Geometry: final body of the model. Coordinates: model frame, mm. A direction names the side the tool comes from. Give positions to 0.01 mm unless a question says otherwise; leave off trailing zeros. Loops run counter-clockwise (first coordinate to the right, second up) from the corner with the lowest first, then second, coordinate; pieces in that order, holes last. Notation, with made-up numbers: (35.25, 23) - (88.25, 23) arc R16 cw to (88.25, 31) - close; hole circle Ø2 at (73.5, 86.25). An arc over 180 degrees is marked (long way). Answer in a Markdown table with one row per item.
from build123d import *

# Parameters (mm, degrees)
F1_DEPTH = 5
F3_DEPTH = 22
F5_D     = 12
F5_DEPTH = 24
F5_TIP   = 3.6051637142
F7_D     = 6
F7_DEPTH = 16
F7_TIP   = 1.8025818571


with BuildPart() as f1:
    # F0 (on Front) → F1 (new body, symmetric)
    with BuildSketch(Plane.XZ):
        Polygon((32, -18), (32, 18), (-32, 18), (-32, -18), (-8, -18), (-8, -27), (8, -27), (8, -18), align=None)
    extrude(amount=F1_DEPTH, both=True)

    # F2 (on face) → F3 (join)
    with BuildSketch(Plane.XZ.offset(5)):
        with BuildLine():
            Line((-27.5, -8), (-32, -8))
            Line((-32, -8), (-32, -18))
            Line((-32, -18), (-8, -18))
            Line((-8, -18), (-8, -27))
            Line((-8, -27), (8, -27))
            Line((8, -27), (8, -18))
            Line((8, -18), (32, -18))
            Line((32, -18), (32, -8))
            Line((32, -8), (27.5, -8))
            ThreePointArc((27.5, -8), (26.0843309615, -7.6449728115), (25.0037292554, -6.6639207823))
            Line((25.0037292554, -6.6639207823), (13.3134439711, 10.8742441722))
            ThreePointArc((13.3134439711, 10.8742441722), (7.5502348479, 16.1065216741), (-5.46e-08, 18))
            ThreePointArc((-5.46e-08, 18), (-7.5502348961, 16.1065216483), (-13.3134439711, 10.8742441722))
            Line((-13.3134439711, 10.8742441722), (-25.0037292554, -6.6639207823))
            ThreePointArc((-25.0037292554, -6.6639207823), (-26.0843309615, -7.6449728115), (-27.5, -8))
        make_face()
    extrude(amount=F3_DEPTH)

    # F5
    with Locations(Plane.XZ.offset(27)):
        with Locations((0, 2)):
            Hole(F5_D / 2, depth=F5_DEPTH)
            with Locations((0, 0, -(F5_DEPTH + F5_TIP / 2))):  # 118° drill point
                Cone(0, F5_D / 2, F5_TIP, mode=Mode.SUBTRACT)

    # F7
    with Locations(Plane(origin=(0, 0, -27), x_dir=(1, 0, 0), z_dir=(0, 0, -1))):
        with Locations((0, 19), (0, 3)):
            Hole(F7_D / 2, depth=F7_DEPTH)
            with Locations((0, 0, -(F7_DEPTH + F7_TIP / 2))):  # 118° drill point
                Cone(0, F7_D / 2, F7_TIP, mode=Mode.SUBTRACT)


solid = f1.part
Q1. Cut plane B-B (z = -14.5). Output: boundary loops of the cut face in (x, y), and give its area (3 significant figures).
Check values:
| item | result |
|---|---|
| outline | (-32, -27) - (32, -27) - (32, 5) - (-32, 5) - close; hole circle Ø6 at (0, -19); hole circle Ø6 at (0, -3) |
| area | 1,990 mm² |
Q2. First-contact query: pin 1 (19 mm diameter, centred on x = -18.5, y = -15, fed in from -Z); pin 2 (5 mm diameter, centred on x = 30.5, y = -19.5, fed in from +Z); pin 3 (1.5 mm diameter, centred on x = -12.5, y = -6.5, fed in from +Z). Flat tips, straight axial feed; report the tip coordinate or a pass-through.
Check values:
| item | result |
|---|---|
| pin 1 | z = -18 |
| pin 2 | z = -8 |
| pin 3 | z = 12.86 |
Q3. Cut plane D-D (z = -21). Output: boundary loops of the cut face in (x, y), and give its area (3 significant figures).
Check values:
| item | result |
|---|---|
| outline | (-8, -27) - (8, -27) - (8, 5) - (-8, 5) - close; hole circle Ø6 at (0, -19); hole circle Ø6 at (0, -3) |
| area | 455 mm² |
Q4. Reachability of faces 1 (the flat face through (-20, -11, -18)), 2 (the flat face through (-19.077, -15.846, 2.228)), 3 (the flat face through (19.24, -15.85, 1.98)) from +Z, -Z, +X, -X, +Y, -Y: full face, straight path, thin tool, end or side. Return the list, or none.
Check values:
| item | result |
|---|---|
| face 1 | -Z, -X, +Y, -Y |
| face 2 | +Z, -X, -Y |
| face 3 | +Z, +X, -Y |
Q5. Material intervals for line 1 along Y through (x, z) = (0, -22); line 2 along X through (y, z) = (-19, -21); line 3 along X through (y, z) = (-19, -17.5), sorted ascending.
Check values:
| item | result |
|---|---|
| line 1 | -27 to -22, -16 to -6, 0 to 5 |
| line 2 | -8 to -3, 3 to 8 |
| line 3 | -32 to -3, 3 to 32 |
Q6. Cut plane A-A (y = -9.5). Output: boundary loops of the cut face in (x, z).
Check values:
| item | result |
|---|---|
| outline | (-32, -18) - (-8, -18) - (-8, -27) - (8, -27) - (8, -18) - (32, -18) - (32, -8) - (27.5, -8) arc R3 cw to (25, -6.66) - (13.31, 10.87) arc R16 ccw to (-13.31, 10.87) - (-25, -6.66) arc R3 cw to (-27.5, -8) - (-32, -8) - close; hole circle Ø12 at (0, 2) |
Q7. Cut plane C-C (x = -19.5). Output: boundary loops of the cut face in (y, z).
Check values:
| item | result |
|---|---|
| outline | (-27, -18) - (5, -18) - (5, 18) - (-5, 18) - (-5, 1.59) - (-27, 1.59) - close |
Q8. Draft query along Z for faces 4 (the flat face through (30, -16, -8)), 5 (the conical face through (-0.226, -0.021, 0.983)), 6 (the flat face through (-8, -11, -22)). Return one class per face: pulls with the +Z half, pulls with the -Z half, needs draft (parallel to the pull), parting line crosses it, or undercut.
Check values:
| item | result |
|---|---|
| face 4 | pulls with the +Z half |
| face 5 | undercut |
| face 6 | needs draft |
